Source: CAD feature listing. Evaluate the final solid. Frame: model axes, mm. Face numbers are marked on the shaded views. Give positions to 0.01 mm unless a question says otherwise; leave off trailing zeros. Loops run counter-clockwise (first coordinate to the right, second up) from the corner with the lowest first, then second, coordinate; pieces in that order, holes last. Notation, with made-up numbers: M 25,71 L 79,71 A30 ccw 79,105 Z; hole C -2,42 d9. An arc over 180 degrees is marked long. Answer in a Markdown table with one row per item.
```python
from build123d import *

# Parameters (mm, degrees)
SKETCH_1_W          = 104
SKETCH_1_H          = 135
EXTRUDE_2_DEPTH     = 5
SKETCH_2_W          = 20
SKETCH_2_H          = 4
SKETCH_2_W_2        = 4
SKETCH_2_H_2        = 20
EXTRUDE_3_DEPTH     = 10
CUT_EXTRUDE_1_REACH = 7
SKETCH_3_W          = 57
SKETCH_3_H          = 15
SKETCH_4_W          = 5
SKETCH_4_H          = 6
EXTRUDE_4_DEPTH     = 15
SKETCH_6_W          = 53
SKETCH_6_H          = 6
EXTRUDE_5_DEPTH     = 7


with BuildPart() as part:
    # 草圖1 → 填料-伸長2 (new body)
    with BuildSketch(Plane.XY):
        with Locations((34.103184984, -53.003221767)):
            Rectangle(SKETCH_1_W, SKETCH_1_H)
    extrude(amount=EXTRUDE_2_DEPTH)

    # 草圖2 → 填料-伸長3 (add)
    with BuildSketch(Plane.XY.offset(5)):
        with Locations((39.103184984, 10.496778233)):
            Rectangle(SKETCH_2_W, SKETCH_2_H)
        with Locations((39.103184984, -112.503221767)):
            Rectangle(SKETCH_2_W, SKETCH_2_H)
        with Locations((83.103184984, -62.503221767)):
            Rectangle(SKETCH_2_W_2, SKETCH_2_H_2)
    extrude(amount=EXTRUDE_3_DEPTH)

    # 草圖3 → 除料-伸長1 (cut, up to next)
    with BuildSketch(Plane.XY.offset(5), mode=Mode.PRIVATE) as cut_extrude_1_sk1:
        with Locations((42.603184984, -97.003221767)):
            Rectangle(SKETCH_3_W, SKETCH_3_H)
    cut_extrude_1_tool1 = extrude(cut_extrude_1_sk1.sketch, amount=-CUT_EXTRUDE_1_REACH, mode=Mode.PRIVATE) & part.part
    add(cut_extrude_1_tool1.solids().sort_by_distance((42.603185, -97.003222, 5))[0], mode=Mode.SUBTRACT)
    # 草圖3 → 除料-伸長1 (cut, up to next)
    with BuildSketch(Plane.XY.offset(5), mode=Mode.PRIVATE) as cut_extrude_1_sk2:
        with Locations((42.603184984, -76.003221767)):
            Rectangle(SKETCH_3_W, SKETCH_3_H)
    cut_extrude_1_tool2 = extrude(cut_extrude_1_sk2.sketch, amount=-CUT_EXTRUDE_1_REACH, mode=Mode.PRIVATE) & part.part
    add(cut_extrude_1_tool2.solids().sort_by_distance((42.603185, -76.003222, 5))[0], mode=Mode.SUBTRACT)
    # 草圖3 → 除料-伸長1 (cut, up to next)
    with BuildSketch(Plane.XY.offset(5), mode=Mode.PRIVATE) as cut_extrude_1_sk3:
        with Locations((42.603184984, -55.003221767)):
            Rectangle(SKETCH_3_W, SKETCH_3_H)
    cut_extrude_1_tool3 = extrude(cut_extrude_1_sk3.sketch, amount=-CUT_EXTRUDE_1_REACH, mode=Mode.PRIVATE) & part.part
    add(cut_extrude_1_tool3.solids().sort_by_distance((42.603185, -55.003222, 5))[0], mode=Mode.SUBTRACT)
    # 草圖3 → 除料-伸長1 (cut, up to next)
    with BuildSketch(Plane.XY.offset(5), mode=Mode.PRIVATE) as cut_extrude_1_sk4:
        with Locations((42.603184984, -34.003221767)):
            Rectangle(SKETCH_3_W, SKETCH_3_H)
    cut_extrude_1_tool4 = extrude(cut_extrude_1_sk4.sketch, amount=-CUT_EXTRUDE_1_REACH, mode=Mode.PRIVATE) & part.part
    add(cut_extrude_1_tool4.solids().sort_by_distance((42.603185, -34.003222, 5))[0], mode=Mode.SUBTRACT)

    # 草圖4 → 填料-伸長4 (add)
    with BuildSketch(Plane.XY.offset(5)):
        with Locations((20.603184984, -44.503221767)):
            Rectangle(SKETCH_4_W, SKETCH_4_H)
        with Locations((78.603184984, -44.503221767)):
            Rectangle(SKETCH_4_W, SKETCH_4_H)
        with Locations((20.603184984, -65.503221767)):
            Rectangle(SKETCH_4_W, SKETCH_4_H)
        with Locations((78.603184984, -65.503221767)):
            Rectangle(SKETCH_4_W, SKETCH_4_H)
        with Locations((20.603184984, -86.503221767)):
            Rectangle(SKETCH_4_W, SKETCH_4_H)
        with Locations((78.603184984, -86.503221767)):
            Rectangle(SKETCH_4_W, SKETCH_4_H)
    extrude(amount=EXTRUDE_4_DEPTH)

    # 草圖6 → 填料-伸長5 (add)
    with BuildSketch(Plane.XY.offset(5)):
        with Locations((49.603184984, -44.503221767)):
            Rectangle(SKETCH_6_W, SKETCH_6_H)
        with Locations((49.603184984, -65.503221767)):
            Rectangle(SKETCH_6_W, SKETCH_6_H)
        with Locations((49.603184984, -86.503221767)):
            Rectangle(SKETCH_6_W, SKETCH_6_H)
    extrude(amount=EXTRUDE_5_DEPTH)


solid = part.part
```
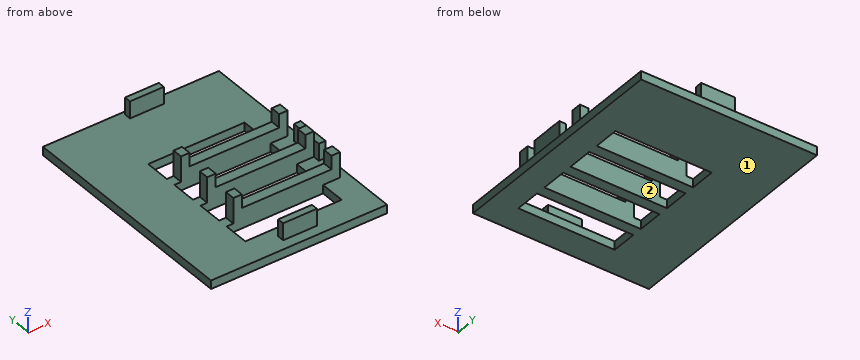
Q1. Ray query, probe 1 along Y at (x, z) = (24.5, 7); probe 2 along X at (y, z) = (-72.5, 3); probe 3 along Y at (x, z) = (49, 13.5). Return the intervals inside material, ascending. Write a range as from..to.
Values follow:
| item | result |
|---|---|
| probe 1 | -89.5..-83.5, -68.5..-62.5, -47.5..-41.5 |
| probe 2 | -17.9..14.1, 71.1..86.1 |
| probe 3 | -114.5..-110.5, 8.5..12.5 |
Q2. Section query A-A (x = 56.5). Output: boundary loops of the cut face in (y, z).
Values follow:
| item | result |
|---|---|
| outline | M -120.5,0 L -104.5,0 L -104.5,5 L -120.5,5 Z; M -89.5,0 L -83.5,0 L -83.5,12 L -89.5,12 Z; M -68.5,0 L -62.5,0 L -62.5,12 L -68.5,12 Z; M -47.5,0 L -41.5,0 L -41.5,12 L -47.5,12 Z; M -26.5,0 L 14.5,0 L 14.5,5 L -26.5,5 Z |
Q3. Section query C-C (y = -57). Output: boundary loops of the cut face in (x, z), plus the area to 3 significant figures.
Values follow:
| item | result |
|---|---|
| outline | M -17.9,0 L 14.1,0 L 14.1,5 L -17.9,5 Z; M 71.1,0 L 86.1,0 L 86.1,5 L 85.1,5 L 85.1,15 L 81.1,15 L 81.1,5 L 71.1,5 Z |
| area | 275 mm^2 |
Q4. Section query D-D (y = -29). Output: boundary loops of the cut face in (x, z).
Values follow:
| item | result |
|---|---|
| outline | M -17.9,0 L 14.1,0 L 14.1,5 L -17.9,5 Z; M 71.1,0 L 86.1,0 L 86.1,5 L 71.1,5 Z |
Q5. Section query B-B (z = 18.25). Output: boundary loops of the cut face in (x, y), plus the area to 3 significant figures.
Values follow:
| item | result |
|---|---|
| outline | M 18.1,-89.5 L 23.1,-89.5 L 23.1,-83.5 L 18.1,-83.5 Z; M 18.1,-68.5 L 23.1,-68.5 L 23.1,-62.5 L 18.1,-62.5 Z; M 18.1,-47.5 L 23.1,-47.5 L 23.1,-41.5 L 18.1,-41.5 Z; M 76.1,-89.5 L 81.1,-89.5 L 81.1,-83.5 L 76.1,-83.5 Z; M 76.1,-68.5 L 81.1,-68.5 L 81.1,-62.5 L 76.1,-62.5 Z; M 76.1,-47.5 L 81.1,-47.5 L 81.1,-41.5 L 76.1,-41.5 Z |
| area | 180 mm^2 |
Q6. Mould query, pull axis Y, two halves, no side actions, for the marked faces 1 and 2. Classes: +Y half, -Y half, draft (parallel to the pull), parting line (faces both ways), or undercut.
Values follow:
| item | result |
|---|---|
| face 1 | draft |
| face 2 | undercut |
Q7. Contact query for flat-ended pins moving along their axis: pin 1 Ø1.2 at (y, z) = (9.5, 11.5) entering from -X; pin 2 Ø4.5 at (x, z) = (82, 8) entering from -Y; pin 3 Ø5 at (y, z) = (-44.5, 14.5) entering from -X; pin 4 Ø1.5 at (x, z) = (40.5, 17) entering from +Y. Output: stop coordinate, or through.
Values follow:
| item | result |
|---|---|
| pin 1 | x = 29.1 |
| pin 2 | y = -89.5 |
| pin 3 | x = 18.1 |
| pin 4 | through |
